Read the model definition and answer for the solid it produces. Units are mm, in the model's axes. Give positions to 0.01 mm unless a question says otherwise; leave off trailing zeros. Order: outer loops, then holes, each group sorted by start corner. A loop starts at its lowest first (then second) coordinate and runs counter-clockwise, first axis right, second up.
```python
from build123d import *

# Parameters (mm, degrees)
SKETCH1_R           = 4
SKETCH1_R_2         = 2
BOSS_EXTRUDE1_DEPTH = 4


with BuildPart() as part:
    # Sketch1 → Boss-Extrude1 (new body)
    with BuildSketch(Plane.XY):
        with BuildLine():
            Line((-40, 0), (-51.681216052, 27.63239388))
            ThreePointArc((-51.681216052, 27.63239388), (-51.692317805, 29.163087351), (-50.617804197, 30.253301209))
            Line((-50.617804197, 30.253301209), (-48.367404943, 31.204626671))
            ThreePointArc((-48.367404943, 31.204626671), (-44.922000222, 31.046750266), (-42.880225189, 28.267021256))
            ThreePointArc((-42.880225189, 28.267021256), (-38.242591008, 22.682316206), (-31.323061762, 24.877013524))
            ThreePointArc((-31.323061762, 24.877013524), (37.768521751, -13.17341128), (-40, 0))
        make_face()
        Circle(SKETCH1_R, mode=Mode.SUBTRACT)
        with Locations((0, 15)):
            Circle(SKETCH1_R_2, mode=Mode.SUBTRACT)
        with Locations((15, 0)):
            Circle(SKETCH1_R_2, mode=Mode.SUBTRACT)
        with Locations((0, -15)):
            Circle(SKETCH1_R_2, mode=Mode.SUBTRACT)
        with Locations((-15, 0)):
            Circle(SKETCH1_R_2, mode=Mode.SUBTRACT)
    extrude(amount=BOSS_EXTRUDE1_DEPTH)


solid = part.part
```
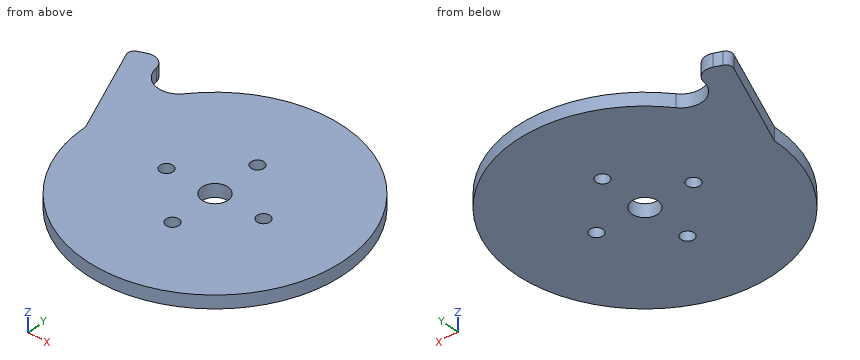
1) Consider L1, parallel to Y at x = 0, z = 1.15; L2, parallel to Y at x = -1.5, z = 3.7; L3, parallel to Y at x = 15, z = 2.1. Determine where each line is inside the solid, lowest interval first.
Final values:
L1: y = -40 to -17, -13 to -4, 4 to 13, 17 to 40
L2: y = -39.97 to -16.32, -13.68 to -3.71, 3.71 to 13.68, 16.32 to 39.97
L3: y = -37.08 to -2, 2 to 37.08
2) The part is cut by section B-B on y = -15. Determine the outline of the cut face in (x, z).
Final values:
outline: (-37.08, 0) - (-2, 0) - (-2, 4) - (-37.08, 4) - close; (2, 0) - (37.08, 0) - (37.08, 4) - (2, 4) - close
3) The part is cut by section C-C on z = 2.45. Determine the outline of the cut face in (x, y).
Final values:
outline: (-51.68, 27.63) - (-40, 0) arc R40 ccw (long way) to (-31.32, 24.88) arc R6.5 cw to (-42.88, 28.27) arc R4 ccw to (-48.37, 31.2) - (-50.62, 30.25) arc R2 ccw to start; hole circle Ø4 at (-15, 0); hole circle Ø8 at (0, 0); hole circle Ø4 at (0, -15); hole circle Ø4 at (0, 15); hole circle Ø4 at (15, 0)
4) Given pin 1 (12 mm diameter, centred on x = -15.5, y = -25.5, fed in from -Z); pin 2 (1.5 mm diameter, centred on x = 24.5, z = 3.5, fed in from -Y); pin 3 (1 mm diameter, centred on x = 26.5, z = 2, fed in from -Y); pin 4 (2 mm diameter, centred on x = 24, z = 1, fed in from -Y), each flat-ended and moving along its own axis, determine where each tip first touches the part or whether it passes through.
Final values:
pin 1: stops at z = 0
pin 2: stops at y = -32.19
pin 3: stops at y = -30.4
pin 4: stops at y = -32.73
5) The part is cut by section A-A on x = 0. Determine the outline of the cut face in (y, z), and give its area (3 significant figures).
Final values:
outline: (-40, 0) - (-17, 0) - (-17, 4) - (-40, 4) - close; (-13, 0) - (-4, 0) - (-4, 4) - (-13, 4) - close; (4, 0) - (13, 0) - (13, 4) - (4, 4) - close; (17, 0) - (40, 0) - (40, 4) - (17, 4) - close
area: 256 mm2
